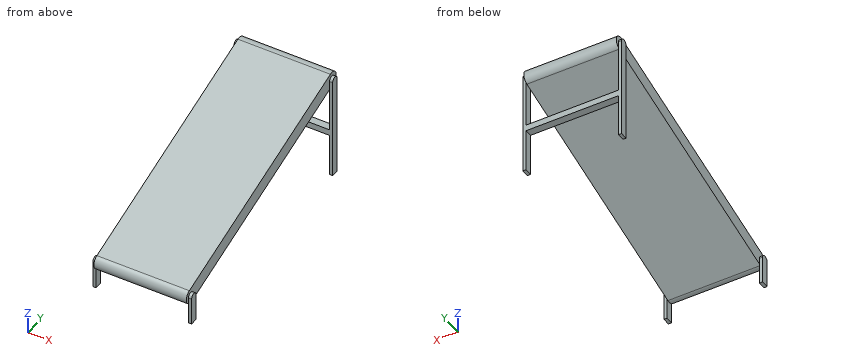
```python
from build123d import *

# Parameters (mm, degrees)
F1_DEPTH = 375
F3_DEPTH = 25
F5_W     = 60
F5_H     = 50
F6_DEPTH = 750


with BuildPart() as f1:
    # F0 (on Right) → F1 (new body, symmetric)
    with BuildSketch(Plane.YZ):
        with BuildLine():
            Line((934.052350761, 890), (-970.652350761, 280))
            ThreePointArc((-970.652350761, 280), (-1009.4934918067, 204.5588589543), (-934.052350761, 165.7177179087))
            Line((-934.052350761, 165.7177179087), (970.652350761, 775.7177179087))
            ThreePointArc((970.652350761, 775.7177179087), (1009.4934918067, 851.1588589543), (934.052350761, 890))
        make_face()
    extrude(amount=F1_DEPTH, both=True)

    # F2 (on face) → F3 (join)
    with BuildSketch(Plane.YZ.offset(375)):
        with BuildLine():
            Line((-982.352350761, 222.8588589543), (-982.352350761, 0))
            Line((-982.352350761, 0), (-922.352350761, 0))
            Line((-922.352350761, 0), (-922.352350761, 222.8588589543))
            ThreePointArc((-922.352350761, 222.8588589543), (-952.352350761, 252.8588589543), (-982.352350761, 222.8588589543))
        make_face()
        with BuildLine():
            Line((922.352350761, 832.8588589543), (922.352350761, 0))
            Line((922.352350761, 0), (982.352350761, 0))
            Line((982.352350761, 0), (982.352350761, 832.8588589543))
            ThreePointArc((982.352350761, 832.8588589543), (952.352350761, 862.8588589543), (922.352350761, 832.8588589543))
        make_face()
    extrude(amount=F3_DEPTH)

    # F4: F1 across plane


with BuildPart() as f1_1:
    add(f1.part)
    add(f1.part.mirror(Plane.YZ))

    # F5 (on face) → F6 (join, through all)
    with BuildSketch(Plane.YZ.offset(-375)):
        with Locations((952.352350761, 375)):
            Rectangle(F5_W, F5_H)
    extrude(amount=F6_DEPTH)


solid = f1_1.part
```
Check sheet for the modelled part. Datum: model origin and axes. Units: mm. Give positions to 0.01 mm unless a question says otherwise; leave off trailing zeros. Order: outer loops, then holes, each group sorted by start corner. A loop starts at its lowest first (then second) coordinate and runs counter-clockwise, first axis right, second up. Notation, with made-up numbers: M -4.5,56.5 L 16.5,56.5 A20 ccw 16.5,78.5 Z; hole C 15.25,80 d3. An arc over 180 degrees is marked long. Answer in a Markdown table with one row per item.
1) Cross-section at B-B, the plane z = 693. Enter the section's corners in (x, y).
Filled sheet:
| item | result |
|---|---|
| outline | M -400,922.35 L -375,922.35 L -375,982.35 L -400,982.35 Z; M -375,318.93 L 375,318.93 L 375,712.37 L -375,712.37 Z; M 375,922.35 L 400,922.35 L 400,982.35 L 375,982.35 Z |
2) Cross-section at D-D, the plane y = 850.5. Enter the section's corners in (x, z).
Filled sheet:
| item | result |
|---|---|
| outline | M -375,737.24 L 375,737.24 L 375,863.24 L -375,863.24 Z |
3) Gauge pin test, flat ends, axial feed: P1, Ø1.5, axis at x = 2.5, y = 126, coming from the -Z side; P2, Ø4, axis at y = 808.5, z = 720.5, coming from the +X side; P3, Ø12.5, axis at x = -382, z = 107.5, coming from the -Y side; P4, Ø5, axis at x = 184.5, y = -167.5, coming from the -Z side. Record the tip position at first contact, or that the pin passes through.
Filled sheet:
| item | result |
|---|---|
| P1 | stops at z = 504.97 |
| P2 | passes through |
| P3 | stops at y = -982.35 |
| P4 | stops at z = 410.41 |
4) Thickness scan on L1, parallel to X at y = -845, z = 243; L2, parallel to Z at x = -258.5, y = 925; L3, parallel to Z at x = -120.5, y = -445. Record the ranges inside material, lowest first. Write a range as [from, to].
Filled sheet:
| item | result |
|---|---|
| L1 | x = [-375, 375] |
| L2 | z = [350, 400], [761.1, 887.1] |
| L3 | z = [322.34, 448.35] |
5) Cross-section at A-A, the plane x = -93. Enter the section's corners in (y, z), plus the area to 3 significant figures.
Filled sheet:
| item | result |
|---|---|
| outline | M -970.65,280 A60 ccw -934.05,165.72 L 970.65,775.72 A60 ccw 934.05,890 Z; M 922.35,350 L 982.35,350 L 982.35,400 L 922.35,400 Z |
| area | 254,000 mm2 |
6) Cross-section at C-C, the plane z = 809.5. Enter the section's corners in (x, y), plus the area to 3 significant figures.
Filled sheet:
| item | result |
|---|---|
| outline | M -400,922.35 L -375,922.35 L -375,682.69 L 375,682.69 L 375,922.35 L 400,922.35 L 400,982.35 L 375,982.35 L 375,1007.62 L -375,1007.62 L -375,982.35 L -400,982.35 Z |
| area | 247,000 mm2 |
